Geometry check sheet. Reference: the model listing, model coordinates, mm. Face numbers are marked on the shaded views. A direction names the side the tool comes from. Give positions to 0.01 mm unless a question says otherwise; leave off trailing zeros. Loops run counter-clockwise (first coordinate to the right, second up) from the corner with the lowest first, then second, coordinate; pieces in that order, holes last. Notation, with made-up numbers: (-18, -9) -> (1, -9) arc R29 cw to (1, 13) -> close; hole circle Ø7 at (-10, 42). An arc over 180 degrees is marked (long way). Answer as a JSON object with one key per item and string values.
from build123d import *

# Parameters (mm, degrees)
BOSS_EXTRUDE1_DEPTH = 1.5
BOSS_EXTRUDE2_DEPTH = 6.5
SKETCH3_R           = 1.5
CUT_EXTRUDE1_DEPTH  = 6.5


with BuildPart() as part:
    # Sketch1 → Boss-Extrude1 (new body)
    with BuildSketch(Plane(origin=(0, 0, 0), x_dir=(1, 0, 0), z_dir=(0, 1, 0))):
        Polygon((-7, 0), (-10, 3), (-10, 35), (0, 35), (0, 3), (-3, 0), align=None)
    extrude(amount=BOSS_EXTRUDE1_DEPTH)

    # Sketch2 → Boss-Extrude2 (add)
    with BuildSketch(Plane.XZ):
        Polygon((-3.25, 0), (-6.75, 0), (-7.75, -1), (-7.75, -10), (-2.25, -10), (-2.25, -1), align=None)
    extrude(amount=BOSS_EXTRUDE2_DEPTH)

    # Sketch3 → Cut-Extrude1 (cut)
    with BuildSketch(Plane(origin=(0, 1.5, 0), x_dir=(1, 0, 0), z_dir=(0, 1, 0))):
        with Locations(Location((-5, 17.5, 0), (0, 0, 270))):
            Circle(SKETCH3_R)
    extrude(amount=-CUT_EXTRUDE1_DEPTH, mode=Mode.SUBTRACT)


solid = part.part
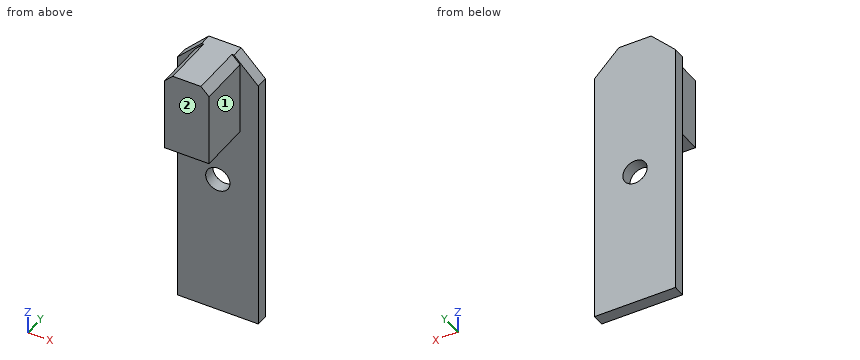
1) Material ranges on line 1 along X through (y, z) = (1, -17.5); line 2 along Y through (x, z) = (-5.5, -16); line 3 along Z through (x, y) = (-2.5, -6), recorded low to high. Write a range as from..to.
Geometry check:
{"line 1": "x = -10..-6.5, -3.5..0", "line 2": "y = 0..1.5", "line 3": "z = -10..-0.75"}
2) Depth check by flat-ended pin: P1, Ø5, axis at x = -7, z = -16, coming from the -Y side; P2, Ø3, axis at y = -0.5, z = -21.5, coming from the +X side; P3, Ø1.6, axis at x = -5, y = -3, coming from the -Z side. Enter the tip coordinate at first touch or a pass-through.
Geometry check:
{"P1": "stops at y = 0", "P2": "stops at x = 0", "P3": "stops at z = -10"}
3) Tool access check on the marked faces 1 and 2. Record the directions out of +Z, -Z, +X, -X, +Y, -Y that give a thin tool (end or side, any length) a straight path to the whole face; none if there is none.
Geometry check:
{"face 1": "+Z, -Z, +X, -Y", "face 2": "+Z, -Z, +X, -X, -Y"}
4) Section check B-B on z = -17.5. Record the cut outline in (x, y), plus the area to 3 significant figures.
Geometry check:
{"outline": "(-10, 0) -> (-6.5, 0) -> (-6.5, 1.5) -> (-10, 1.5) -> close; (-3.5, 0) -> (0, 0) -> (0, 1.5) -> (-3.5, 1.5) -> close", "area": "10.5 mm2"}
5) Section check A-A on x = -5. Record the cut outline in (y, z), plus the area to 3 significant figures.
Geometry check:
{"outline": "(-6.5, -10) -> (0, -10) -> (0, -16) -> (1.5, -16) -> (1.5, 0) -> (-6.5, 0) -> close; (0, -35) -> (1.5, -35) -> (1.5, -19) -> (0, -19) -> close", "area": "113 mm2"}
6) Section check D-D on z = -5.5. Record the cut outline in (x, y), plus the area to 4 significant figures.
Geometry check:
{"outline": "(-10, 0) -> (-7.75, 0) -> (-7.75, -6.5) -> (-2.25, -6.5) -> (-2.25, 0) -> (0, 0) -> (0, 1.5) -> (-10, 1.5) -> close", "area": "50.75 mm2"}
7) Section check C-C on y = -2.5. Record the cut outline in (x, z).
Geometry check:
{"outline": "(-7.75, -10) -> (-2.25, -10) -> (-2.25, -1) -> (-3.25, 0) -> (-6.75, 0) -> (-7.75, -1) -> close"}
